For this review, take the finished solid that the model builds, in its own axes (mm). Face numbers are marked on the shaded views. A direction names the side the tool comes from. Coordinates: 2 decimals unless noted, no trailing zeros. Write each loop counter-clockwise with the first axis right and the second up, starting at its lowest first coordinate (ties: lowest second). Pieces come first, ordered by that corner, then holes. Notation, with made-up numbers: (25.5, -8) -> (30.5, -8) arc R12 cw to (30.5, 11) -> close; hole circle Ø4 at (29, -16.5). An arc over 180 degrees is marked (long way). One line per item, written item: value. Start each with the question number.
1) Machinability: for the marked faces 1 and 2, which of the approach directions +Z, -Z, +X, -X, +Y, -Y give a long, thin tool a straight path to every point of the face, cutting with its end or side? Answer none if there is none.
2) For probe 1 along Z at (x, y) = (7.3, -50.8); probe 2 along Y at (x, z) = (2.25, 21); probe 3 along Y at (x, z) = (4, 18), list the stretches that pass through material, from the lowest coordinate up. Write a range as from..to.
3) Add section B-B (x = 4.25). State the section outline as (y, z) points (1 decimal), and give its area (3 significant figures).
4) Add section C-C (z = 25). State the section outline as (x, y) points (3 decimals).
5) Add section D-D (z = 57). State the section outline as (x, y) points.
6) For pin 1 Ø2 at (x, y) = (8, -66.5) entering from +Z; pin 2 Ø3.5 at (y, z) = (-53.5, 22) entering from -X; pin 3 Ø5.5 at (y, z) = (-54, 64.5) entering from +X; pin 4 Ø4 at (y, z) = (-76.2, 20.64) entering from -X, all flat-tipped, find the tip position at first contact; note any pin that passes through.
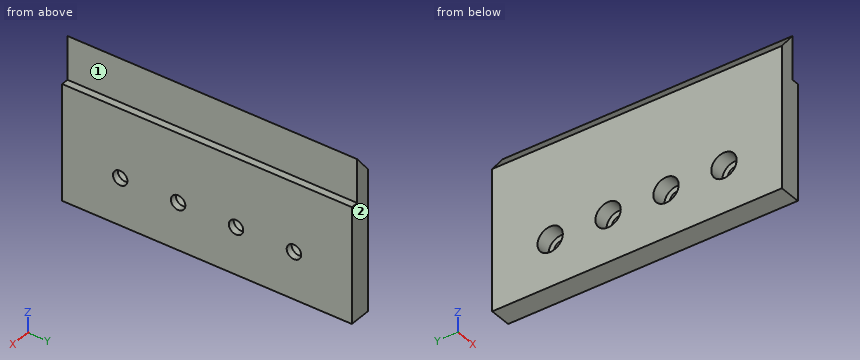
from build123d import *

# Parameters (mm, degrees)
F1_DEPTH = 127
F3_DEPTH = 25.4
F4_R     = 5.55625
F5_DEPTH = 6.604


with BuildPart() as f1:
    # F0 (on Front) → F1 (new body)
    with BuildSketch(Plane.XZ):
        Polygon((0, 61.9125), (0, 0), (9.525, 0), (9.525, 50.8), (6.35, 50.8), (6.35, 69.85), align=None)
    extrude(amount=F1_DEPTH)

    # F2 (on face) → F3 (cut)
    with BuildSketch(Plane(origin=(0, 0, 0), x_dir=(0, -1, 0), z_dir=(-1, 0, 0))):
        with BuildLine():
            ThreePointArc((98.425, 20.6375), (101.6, 17.4625), (104.775, 20.6375))
            Line((104.775, 20.6375), (98.425, 20.6375))
        make_face()
        with BuildLine():
            Line((98.425, 20.6375), (104.775, 20.6375))
            ThreePointArc((104.775, 20.6375), (101.6, 23.8125), (98.425, 20.6375))
        make_face()
        with BuildLine():
            ThreePointArc((22.225, 20.6375), (25.4, 17.4625), (28.575, 20.6375))
            Line((28.575, 20.6375), (22.225, 20.6375))
        make_face()
        with BuildLine():
            Line((22.225, 20.6375), (28.575, 20.6375))
            ThreePointArc((28.575, 20.6375), (25.4, 23.8125), (22.225, 20.6375))
        make_face()
        with BuildLine():
            ThreePointArc((47.625, 20.6375), (50.8, 17.4625), (53.975, 20.6375))
            Line((53.975, 20.6375), (47.625, 20.6375))
        make_face()
        with BuildLine():
            Line((47.625, 20.6375), (53.975, 20.6375))
            ThreePointArc((53.975, 20.6375), (50.8, 23.8125), (47.625, 20.6375))
        make_face()
        with BuildLine():
            ThreePointArc((73.025, 20.6375), (76.2, 17.4625), (79.375, 20.6375))
            Line((79.375, 20.6375), (73.025, 20.6375))
        make_face()
        with BuildLine():
            Line((73.025, 20.6375), (79.375, 20.6375))
            ThreePointArc((79.375, 20.6375), (76.2, 23.8125), (73.025, 20.6375))
        make_face()
    extrude(amount=-F3_DEPTH, mode=Mode.SUBTRACT)

    # F4 (on face) → F5 (cut)
    with BuildSketch(Plane(origin=(0, 0, 0), x_dir=(0, -1, 0), z_dir=(-1, 0, 0))):
        with Locations((101.6, 20.6375)):
            Circle(F4_R)
        with Locations((76.2, 20.6375)):
            Circle(F4_R)
        with Locations((50.8, 20.6375)):
            Circle(F4_R)
        with Locations((25.4, 20.6375)):
            Circle(F4_R)
    extrude(amount=-F5_DEPTH, mode=Mode.SUBTRACT)


solid = f1.part
Numbers:
1. face 1: +Z, +X, +Y, -Y
1. face 2: +Z, -Z, +X, -X, +Y
2. probe 1: 0..17.46, 23.81..50.8
2. probe 2: -127..-107.14, -96.06..-81.74, -70.66..-56.34, -45.26..-30.94, -19.86..0
2. probe 3: -127..-106.49, -96.71..-81.09, -71.31..-55.69, -45.91..-30.29, -20.51..0
3. outline: (-127, 0) -> (0, 0) -> (0, 67.2) -> (-127, 67.2) -> close; hole circle Ø11.1 at (-101.6, 20.6); hole circle Ø11.1 at (-76.2, 20.6); hole circle Ø11.1 at (-50.8, 20.6); hole circle Ø11.1 at (-25.4, 20.6)
3. area: 8,150 mm²
4. outline: (0, -127) -> (9.525, -127) -> (9.525, 0) -> (0, 0) -> (0, -21.959) -> (6.604, -21.959) -> (6.604, -28.841) -> (0, -28.841) -> (0, -47.359) -> (6.604, -47.359) -> (6.604, -54.241) -> (0, -54.241) -> (0, -72.759) -> (6.604, -72.759) -> (6.604, -79.641) -> (0, -79.641) -> (0, -98.159) -> (6.604, -98.159) -> (6.604, -105.041) -> (0, -105.041) -> close
5. outline: (0, -127) -> (6.35, -127) -> (6.35, 0) -> (0, 0) -> close
6. pin 1: z = 50.8
6. pin 2: x = 6.6
6. pin 3: x = 6.35
6. pin 4: through
